```python
from build123d import *

# Parameters (mm, degrees)
BOSS_EXTRUDE1_DEPTH = 2.54
CUT_EXTRUDE1_START  = -2.54
CUT_EXTRUDE1_DEPTH  = 2.54
CIRPATTERN1_COUNT   = 27
CIRPATTERN1_ANGLE   = 65
FILLET1_R           = 3.048


with BuildPart() as part:
    # Sketch1 → Boss-Extrude1 (new body)
    with BuildSketch(Plane(origin=(0, 0, 0), x_dir=(0, 0, -1), z_dir=(1, 0, 0))):
        with BuildLine():
            ThreePointArc((-43.381076299, 12.030901448), (11.033243319, 22.702964816), (58.576421759, -5.83573347))
            add(Edge.make_bspline(
                [(-36.400312003, -2.96377669), (3.456833979, 27.156600716), (58.576421759, -5.83573347)],
                knots=[0, 0, 0, 1, 1, 1], degree=2))
            ThreePointArc((-36.400312003, -2.96377669), (-42.843357456, -7.694652529), (-49.414438561, -12.246016505))
            ThreePointArc((-49.414438561, -12.246016505), (-52.563618606, -12.471871328), (-54.350611077, -9.868987685))
            ThreePointArc((-54.350611077, -9.868987685), (-51.929499525, 2.615525346), (-43.381076299, 12.030901448))
        make_face()
    extrude(amount=BOSS_EXTRUDE1_DEPTH)

    # Sketch2 → Cut-Extrude1 (cut)
    with BuildSketch(Plane(origin=(2.54, 0, 0), x_dir=(0, 0, -1), z_dir=(1, 0, 0)).offset(CUT_EXTRUDE1_START)):
        with BuildLine():
            ThreePointArc((25.551250128, 18.666636018), (25.832723904, 19.021035399), (25.93313959, 19.462332462))
            ThreePointArc((25.93313959, 19.462332462), (24.821637158, 20.47810228), (23.909811979, 19.279853215))
            ThreePointArc((23.909811989, 19.279853244), (24.732270015, 18.977899406), (25.55125014, 18.666636047))
        make_face()
        with BuildLine():
            ThreePointArc((25.55125014, 18.666636047), (24.732270015, 18.977899406), (23.909811989, 19.279853244))
            ThreePointArc((23.909811979, 19.279853215), (24.556324155, 18.506933739), (25.551250128, 18.666636018))
        make_face()
    cut_extrude1 = extrude(amount=CUT_EXTRUDE1_DEPTH, mode=Mode.SUBTRACT)

    # CirPattern1: Cut-Extrude1 ×27 about axis
    cirpattern1_axis = Axis((0, -53.378286458, 2.29893888), (-1, 0, 0))
    for i in range(1, CIRPATTERN1_COUNT):
        add(cut_extrude1.rotate(cirpattern1_axis, i * CIRPATTERN1_ANGLE / (CIRPATTERN1_COUNT - 1)), mode=Mode.SUBTRACT)

    # Fillet1
    # the kernel refuses this fillet: 3.048 mm, written as the material it takes off along each edge
    with BuildSketch(Plane(origin=(5.330131359, -4.91064789, -57.842493504), x_dir=(0, -0.7831380255895678, -0.6218479178027966), z_dir=(-1, 0, 0)), Plane(origin=(5.330131359, 18.666635995, -25.5512501), x_dir=(0, -0.3672934659287651, -0.9301051069024593), z_dir=(-1, 0, 0)), Plane(origin=(5.330131359, 17.383257012, -28.667298272), x_dir=(0, -0.40751449888321617, -0.913198736968006), z_dir=(-1, 0, 0)), Plane(origin=(5.330131359, 15.965179408, -31.724400451), x_dir=(0, -0.4469598048274426, -0.8945540413349069), z_dir=(-1, 0, 0)), Plane(origin=(5.330131359, 14.415102576, -34.71673727), x_dir=(0, -0.48555429737964134, -0.8742065112410012), z_dir=(-1, 0, 0)), Plane(origin=(5.330131359, 12.735977175, -37.638612645), x_dir=(0, -0.5232245097296833, -0.8521948793662941), z_dir=(-1, 0, 0)), Plane(origin=(5.330131359, 10.930999516, -40.484464621), x_dir=(0, -0.5598987344873042, -0.8285610461031312), z_dir=(-1, 0, 0)), Plane(origin=(5.330131359, 9.003605475, -43.248875957), x_dir=(0, -0.5955071601812754, -0.8033499997963732), z_dir=(-1, 0, 0)), Plane(origin=(5.330131359, 6.957463958, -45.926584439), x_dir=(0, -0.6299820041494215, -0.776609731105578), z_dir=(-1, 0, 0)), Plane(origin=(5.330131359, 4.79646991, -48.512492896), x_dir=(0, -0.663257641566846, -0.7483911416520008), z_dir=(-1, 0, 0)), Plane(origin=(5.330131359, 2.524736907, -51.001678904), x_dir=(0, -0.6952707303664444, -0.7187479471245193), z_dir=(-1, 0, 0)), Plane(origin=(5.330131359, 0.146589322, -53.389404158), x_dir=(0, -0.7259603318141797, -0.6877365750287285), z_dir=(-1, 0, 0)), Plane(origin=(5.330131359, -2.333445906, -55.671123485), x_dir=(0, -0.7552680265094119, -0.6554160572739871), z_dir=(-1, 0, 0))) as fillet1_piece_1:
        with BuildLine():
            CenterArc((1.094032194, 3.047920456), FILLET1_R, 240.878460026, 29.535478311)
            ThreePointArc((-0.389319175, 0.385220188), (-0.168317676, 0.2192323), (0, 0))
            ThreePointArc((0, 0), (0.558026272, -0.002015763), (1.116052544, 0))
        make_face()
    extrude(amount=8.120262718, mode=Mode.SUBTRACT)
    with BuildSketch(Plane(origin=(-2.790131315, 19.27985318, -23.909811985), x_dir=(0, -0.8996941201267986, -0.43652089321046916), z_dir=(1, 0, 0)), Plane(origin=(-2.790131315, 18.067489074, -27.0541706), x_dir=(0, -0.917878584614337, -0.39686131570912947), z_dir=(1, 0, 0)), Plane(origin=(-2.790131315, 16.719123874, -30.142653902), x_dir=(0, -0.9343158150472597, -0.35644629013720247), z_dir=(1, 0, 0)), Plane(origin=(-2.790131315, 15.23732427, -33.169382789), x_dir=(0, -0.9489745222231959, -0.3153527487929306), z_dir=(1, 0, 0)), Plane(origin=(-2.790131315, 13.62491095, -36.12859571), x_dir=(0, -0.9618268024599005, -0.27365891556783495), z_dir=(1, 0, 0)), Plane(origin=(-2.790131315, 11.884953236, -39.014659634), x_dir=(0, -0.9728481907114557, -0.23144415704322063), z_dir=(1, 0, 0)), Plane(origin=(-2.790131315, 10.020763236, -41.822080775), x_dir=(0, -0.982017707138919, -0.18878883141123673), z_dir=(1, 0, 0)), Plane(origin=(-2.790131315, 8.035889542, -44.545515048), x_dir=(0, -0.9893178970466047, -0.1457741355086141), z_dir=(1, 0, 0)), Plane(origin=(-2.790131315, 5.934110473, -47.179778241), x_dir=(0, -0.9947348641081103, -0.10248195025378501), z_dir=(1, 0, 0)), Plane(origin=(-2.790131315, 3.719426885, -49.719855883), x_dir=(0, -0.9982582968187538, -0.05899468478194456), z_dir=(1, 0, 0)), Plane(origin=(-2.790131315, -1.031583847, -54.498302279), x_dir=(0, -0.9996013481872734, 0.028233751117859005), z_dir=(1, 0, 0)), Plane(origin=(-2.790131315, -3.558867172, -56.72757499), x_dir=(0, -0.9974184102705359, 0.07180887726038374), z_dir=(1, 0, 0))) as fillet1_piece_2:
        with BuildLine():
            CenterArc((1.366088814, -2.936073381), FILLET1_R, 105.575244384, 29.535478311)
            ThreePointArc((-0.793333618, -0.784980924), (-0.398084606, -0.391057579), (0, 0))
            ThreePointArc((0, 0), (0.273844853, -0.037451811), (0.547689705, 0))
        make_face()
    extrude(amount=8.120262631, mode=Mode.SUBTRACT)
    with BuildSketch(Plane(origin=(-2.790131315, 1.396054555, -52.160912793), x_dir=(0, 0.6999264755180646, 0.7142149038411757), z_dir=(1, 0, 0))) as fillet1_piece_3:
        with BuildLine():
            CenterArc((1.094032194, 3.047920456), FILLET1_R, 240.878460026, 29.535478311)
            ThreePointArc((-0.389319175, 0.385220188), (-0.168317676, 0.2192323), (0, 0))
            ThreePointArc((0, 0), (0.558026272, -0.002015763), (1.116052544, 0))
        make_face()
    extrude(amount=8.120262631, mode=Mode.SUBTRACT)


solid = part.part
```
The model under review builds one solid part; all positions refer to its coordinate system, in mm. Round coordinates to 2 decimals unless told otherwise and drop trailing zeros. Loops run counter-clockwise (first coordinate to the right, second up) from the corner with the lowest first, then second, coordinate; pieces in that order, holes last. Notation, with made-up numbers: (57, -35.75) -> (79, -35.75) arc R5 cw to (79, -26.75) -> close; hole circle Ø1 at (-8.5, 75.25). An arc over 180 degrees is marked (long way). Answer as a JSON object with one key per item and string values. Group by question number.
1) We need section A-A on y = -7.5. Write out the cut boundary in (x, z).
2) For line 1 (Z direction, x = 0.85, y = 3); line 2 (Z direction, x = 1.7, y = 4.5); line 3 (Z direction, x = 1.1, y = 16), list the stretches that pass through material, from the lowest coordinate up. Write a range as [from, to].
3) For pin 1 Ø1.5 at (x, z) = (1, 41) entering from -Y; pin 2 Ø1 at (x, y) = (1.5, 16.5) entering from -Z, all flat-tipped, find the tip position at first contact; note any pin that passes through.
4) Mouldability with a two-part tool opening along Z and no side actions: class faces 1 (the face through (1.25, -7.63, 42.75)), 2 (the face through (0, 13, 10)), 3 (the face through (1.25, 2.45, 52.01)) as released by +Z, released by -Z, zero draft, split by the parting line, or undercut.
Result set:
{
 "1": {"outline": "(0, 42.57) -> (2.54, 42.57) -> (2.54, 54.42) -> (0, 54.42) -> close"},
 "2": {"line 1": "[-49.83, -41.57], [27.27, 51.73]", "line 2": "[-48.7, -37.99], [24.41, 50.88]", "line 3": "[-30.54, 36.25]"},
 "3": {"pin 1": "y = -6.91", "pin 2": "z = -30.54"},
 "4": {"face 1": "undercut", "face 2": "zero draft", "face 3": "released by +Z"}
}
